Model file for the job. Use its own axes, mm. Face numbers are marked on the shaded views. A direction names the side the tool comes from. Round coordinates to 2 decimals unless told otherwise and drop trailing zeros. Loops run counter-clockwise (first coordinate to the right, second up) from the corner with the lowest first, then second, coordinate; pieces in that order, holes last. Notation, with made-up numbers: (44.25, -33) -> (48.25, -33) arc R5 ccw to (48.25, -26) -> close; hole circle Ø7 at (36.5, -7.5). An arc over 180 degrees is marked (long way). Use a Markdown table: item, result. Add a question column.
```python
from build123d import *

# Parameters (mm, degrees)
F0_W     = 76.2
F0_H     = 38.1
F0_R     = 3.9040723684
F0_W_2   = 0.6455261652
F0_H_2   = 4.2599751749
F0_H_3   = 6.0485428542
F0_R_2   = 3.8989
F1_DEPTH = 12.7


with BuildPart() as f1:
    # F0 (on Top) → F1 (new body)
    with BuildSketch(Plane.XY):
        Rectangle(F0_W, F0_H)
        Polygon((5.4683112539, -8.3463666961), (4.0425748882, -11.8080461533), (0.725272804, -13.5434007948), (-2.9313924856, -12.7404388974), (-5.2164266525, -9.774875257), (-5.0606368145, -6.0343300593), (-2.5369187683, -3.269045974), (1.1738517643, -2.7729301572), (4.3353640105, -4.7781207134), align=None, mode=Mode.SUBTRACT)
        with Locations((-14.1024813056, 6.9073382765)):
            Circle(F0_R, mode=Mode.SUBTRACT)
        Polygon((-31.2197456793, 14.5646184978), (-32.5964540855, 12.8382807598), (-34.8045229299, 12.8382807598), (-36.1812313362, 14.5646184978), (-35.6898897947, 16.7173264462), (-33.7004885077, 17.6753716126), (-31.7110872208, 16.7173264462), align=None, mode=Mode.SUBTRACT)
        with Locations((-1.035253305, 14.0512490247)):
            Rectangle(F0_W_2, F0_H_2, mode=Mode.SUBTRACT)
        Polygon((-4.533408102, 12.5120609141), (-4.533408102, 11.9212614372), (-7.7013370861, 11.9212614372), (-7.7013370861, 17.60413051), (-4.533408102, 17.60413051), (-4.533408102, 17.0170623983), (-7.0408854604, 17.0170623983), (-7.0408854604, 15.1862059144), (-4.6851502834, 15.1862059144), (-4.6851502834, 14.6028691678), (-7.0408854604, 14.6028691678), (-7.0408854604, 12.5120609141), align=None, mode=Mode.SUBTRACT)
        with Locations((-3.0489466797, 14.9455328644)):
            Rectangle(F0_W_2, F0_H_3, mode=Mode.SUBTRACT)
        with BuildLine():
            add(Edge.make_bspline(
                [(-1.3039115934, 17.0108434565), (-1.412743076, 17.1178092565), (-1.412743076, 17.3354722216)],
                knots=[0, 0, 0, 1, 1, 1], degree=2))
            add(Edge.make_bspline(
                [(-1.412743076, 17.3354722216), (-1.412743076, 17.5568665519), (-1.3039115934, 17.6601009868)],
                knots=[0, 0, 0, 1, 1, 1], degree=2))
            add(Edge.make_bspline(
                [(-1.3039115934, 17.6601009868), (-1.1950801108, 17.7633354217), (-1.0309000457, 17.7633354217)],
                knots=[0, 0, 0, 1, 1, 1], degree=2))
            add(Edge.make_bspline(
                [(-1.0309000457, 17.7633354217), (-0.8754264992, 17.7633354217), (-0.7628636515, 17.6582353042)],
                knots=[0, 0, 0, 1, 1, 1], degree=2))
            add(Edge.make_bspline(
                [(-0.7628636515, 17.6582353042), (-0.6503008038, 17.5531351868), (-0.6503008038, 17.3354722216)],
                knots=[0, 0, 0, 1, 1, 1], degree=2))
            add(Edge.make_bspline(
                [(-0.6503008038, 17.3354722216), (-0.6503008038, 17.1178092565), (-0.7628636515, 17.0108434565)],
                knots=[0, 0, 0, 1, 1, 1], degree=2))
            add(Edge.make_bspline(
                [(-0.7628636515, 17.0108434565), (-0.8754264992, 16.9038776565), (-1.0309000457, 16.9038776565)],
                knots=[0, 0, 0, 1, 1, 1], degree=2))
            add(Edge.make_bspline(
                [(-1.0309000457, 16.9038776565), (-1.1950801108, 16.9038776565), (-1.3039115934, 17.0108434565)],
                knots=[0, 0, 0, 1, 1, 1], degree=2))
        make_face(mode=Mode.SUBTRACT)
        with Locations((13.814676553, 7.1951444261)):
            Circle(F0_R_2, mode=Mode.SUBTRACT)
        with BuildLine():
            Line((3.7539538223, 11.9212614372), (3.275095299, 11.9212614372))
            Line((3.275095299, 11.9212614372), (3.1469850967, 12.5282301629))
            Line((3.1469850967, 12.5282301629), (3.1158903874, 12.5282301629))
            add(Edge.make_bspline(
                [(3.1158903874, 12.5282301629), (2.7974805641, 12.127730307), (2.4809364233, 11.9853165384)],
                knots=[0, 0, 0, 1, 1, 1], degree=2))
            add(Edge.make_bspline(
                [(2.4809364233, 11.9853165384), (2.1643922826, 11.8429027698), (1.6892651244, 11.8429027698)],
                knots=[0, 0, 0, 1, 1, 1], degree=2))
            add(Edge.make_bspline(
                [(1.6892651244, 11.8429027698), (1.0561768429, 11.8429027698), (0.6967220033, 12.1700191117)],
                knots=[0, 0, 0, 1, 1, 1], degree=2))
            add(Edge.make_bspline(
                [(0.6967220033, 12.1700191117), (0.3372671638, 12.4971354536), (0.3372671638, 13.0991290258)],
                knots=[0, 0, 0, 1, 1, 1], degree=2))
            add(Edge.make_bspline(
                [(0.3372671638, 13.0991290258), (0.3372671638, 14.3889375678), (2.4007120733, 14.4511269864)],
                knots=[0, 0, 0, 1, 1, 1], degree=2))
            Line((2.4007120733, 14.4511269864), (3.1233531176, 14.4747589655))
            Line((3.1233531176, 14.4747589655), (3.1233531176, 14.7396858887))
            add(Edge.make_bspline(
                [(3.1233531176, 14.7396858887), (3.1233531176, 15.2409326028), (2.9081777292, 15.4797399702)],
                knots=[0, 0, 0, 1, 1, 1], degree=2))
            add(Edge.make_bspline(
                [(2.9081777292, 15.4797399702), (2.6930023408, 15.7185473377), (2.2178751826, 15.7185473377)],
                knots=[0, 0, 0, 1, 1, 1], degree=2))
            add(Edge.make_bspline(
                [(2.2178751826, 15.7185473377), (1.6855337593, 15.7185473377), (1.0138880383, 15.3926747842)],
                knots=[0, 0, 0, 1, 1, 1], degree=2))
            Line((1.0138880383, 15.3926747842), (0.8148818987, 15.886458768))
            add(Edge.make_bspline(
                [(0.8148818987, 15.886458768), (1.1295603569, 16.056857775), (1.5045625511, 16.153873268)],
                knots=[0, 0, 0, 1, 1, 1], degree=2))
            add(Edge.make_bspline(
                [(1.5045625511, 16.153873268), (1.8795647453, 16.250888761), (2.2576764105, 16.250888761)],
                knots=[0, 0, 0, 1, 1, 1], degree=2))
            add(Edge.make_bspline(
                [(2.2576764105, 16.250888761), (3.0188748943, 16.250888761), (3.3864143583, 15.913200218)],
                knots=[0, 0, 0, 1, 1, 1], degree=2))
            add(Edge.make_bspline(
                [(3.3864143583, 15.913200218), (3.7539538223, 15.5755116749), (3.7539538223, 14.8292386515)],
                knots=[0, 0, 0, 1, 1, 1], degree=2))
            Line((3.7539538223, 14.8292386515), (3.7539538223, 11.9212614372))
        make_face(mode=Mode.SUBTRACT)
        with BuildLine():
            add(Edge.make_bspline(
                [(7.5636776065, 13.7869439956), (7.8298483182, 13.5070916119), (7.8298483182, 13.0829597769)],
                knots=[0, 0, 0, 1, 1, 1], degree=2))
            add(Edge.make_bspline(
                [(7.8298483182, 13.0829597769), (7.8298483182, 12.488428935), (7.3870596577, 12.1656658524)],
                knots=[0, 0, 0, 1, 1, 1], degree=2))
            add(Edge.make_bspline(
                [(7.3870596577, 12.1656658524), (6.9442709971, 11.8429027698), (6.1432712854, 11.8429027698)],
                knots=[0, 0, 0, 1, 1, 1], degree=2))
            add(Edge.make_bspline(
                [(6.1432712854, 11.8429027698), (5.2962514039, 11.8429027698), (4.8223680341, 12.1115610582)],
                knots=[0, 0, 0, 1, 1, 1], degree=2))
            Line((4.8223680341, 12.1115610582), (4.8223680341, 12.7098232652))
            add(Edge.make_bspline(
                [(4.8223680341, 12.7098232652), (5.129583762, 12.5543497187), (5.4809539772, 12.4654188501)],
                knots=[0, 0, 0, 1, 1, 1], degree=2))
            add(Edge.make_bspline(
                [(5.4809539772, 12.4654188501), (5.8323241923, 12.3764879815), (6.1594405342, 12.3764879815)],
                knots=[0, 0, 0, 1, 1, 1], degree=2))
            add(Edge.make_bspline(
                [(6.1594405342, 12.3764879815), (6.6644186134, 12.3764879815), (6.9361863727, 12.5375585757)],
                knots=[0, 0, 0, 1, 1, 1], degree=2))
            add(Edge.make_bspline(
                [(6.9361863727, 12.5375585757), (7.2079541321, 12.6986291699), (7.2079541321, 13.0294768769)],
                knots=[0, 0, 0, 1, 1, 1], degree=2))
            add(Edge.make_bspline(
                [(7.2079541321, 13.0294768769), (7.2079541321, 13.2782345514), (6.9927787437, 13.4548525002)],
                knots=[0, 0, 0, 1, 1, 1], degree=2))
            add(Edge.make_bspline(
                [(6.9927787437, 13.4548525002), (6.7776033553, 13.6314704491), (6.1507340156, 13.8727653933)],
                knots=[0, 0, 0, 1, 1, 1], degree=2))
            add(Edge.make_bspline(
                [(6.1507340156, 13.8727653933), (5.5562031737, 14.0941597236), (5.3055798167, 14.2595835771)],
                knots=[0, 0, 0, 1, 1, 1], degree=2))
            add(Edge.make_bspline(
                [(5.3055798167, 14.2595835771), (5.0549564597, 14.4250074306), (4.932443305, 14.6345857713)],
                knots=[0, 0, 0, 1, 1, 1], degree=2))
            add(Edge.make_bspline(
                [(4.932443305, 14.6345857713), (4.8099301504, 14.844164112), (4.8099301504, 15.1352105911)],
                knots=[0, 0, 0, 1, 1, 1], degree=2))
            add(Edge.make_bspline(
                [(4.8099301504, 15.1352105911), (4.8099301504, 15.6563579191), (5.2340619853, 15.9579765994)],
                knots=[0, 0, 0, 1, 1, 1], degree=2))
            add(Edge.make_bspline(
                [(5.2340619853, 15.9579765994), (5.6581938202, 16.2595952796), (6.395760325, 16.2595952796)],
                knots=[0, 0, 0, 1, 1, 1], degree=2))
            add(Edge.make_bspline(
                [(6.395760325, 16.2595952796), (7.0835752948, 16.2595952796), (7.7415393437, 15.9797428959)],
                knots=[0, 0, 0, 1, 1, 1], degree=2))
            Line((7.7415393437, 15.9797428959), (7.5114384949, 15.4548642028))
            add(Edge.make_bspline(
                [(7.5114384949, 15.4548642028), (6.8708874832, 15.7185473377), (6.3497401552, 15.7185473377)],
                knots=[0, 0, 0, 1, 1, 1], degree=2))
            add(Edge.make_bspline(
                [(6.3497401552, 15.7185473377), (5.8907822458, 15.7185473377), (5.657571926, 15.5748897807)],
                knots=[0, 0, 0, 1, 1, 1], degree=2))
            add(Edge.make_bspline(
                [(5.657571926, 15.5748897807), (5.4243616062, 15.4312322237), (5.4243616062, 15.1787431842)],
                knots=[0, 0, 0, 1, 1, 1], degree=2))
            add(Edge.make_bspline(
                [(5.4243616062, 15.1787431842), (5.4243616062, 15.0071003888), (5.5120486865, 14.8870748109)],
                knots=[0, 0, 0, 1, 1, 1], degree=2))
            add(Edge.make_bspline(
                [(5.5120486865, 14.8870748109), (5.5997357667, 14.7670492329), (5.7937667528, 14.6582177504)],
                knots=[0, 0, 0, 1, 1, 1], degree=2))
            add(Edge.make_bspline(
                [(5.7937667528, 14.6582177504), (5.9877977389, 14.5493862678), (6.5400397762, 14.342917398)],
                knots=[0, 0, 0, 1, 1, 1], degree=2))
            add(Edge.make_bspline(
                [(6.5400397762, 14.342917398), (7.2975068949, 14.0667963794), (7.5636776065, 13.7869439956)],
                knots=[0, 0, 0, 1, 1, 1], degree=2))
        make_face(mode=Mode.SUBTRACT)
    extrude(amount=F1_DEPTH)


solid = f1.part
```
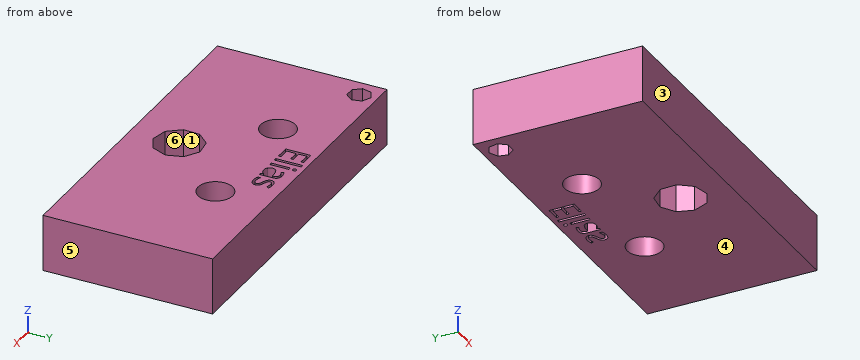
1) Pull direction Y, two halves, no side cores. Call the marked faces 1, 2, 3 and 4: +Y half, -Y half, draft (parallel to the pull), parting line (faces both ways), or undercut.
2) Cut at B-B on y = -11. Write the cut outline in (x, z), and give its area (3 significant figures).
3) Tool access for the marked faces 5 and 6: list every direction of +Z, -Z, +X, -X, +Y, -Y with a clear straight run to the whole face (end or side of a thin tool).
4) Cut at A-A on y = 8.5. Write the cut outline in (x, z), and give its area (3 significant figures).
5) Pin check, flat tips, straight feed: pin 1 Ø4.5 at (x, y) = (-14.1, 6.91) entering from +Z; pin 2 Ø8 at (x, y) = (13, 3.5) entering from -Z. Stop position of each tip, or through.
6) Cut at C-C on z = 8.5. Count the separate pieces of the cut face and the enclosed holes in it, and give its area (3 significant figures).
7) Wall check: probe 1 along X at (y, z) = (7, 5.25); probe 2 along X at (y, z) = (17.5, 2); probe 3 along Y at (x, z) = (-14, 5). Give the ranges that are in metal, low to high. Write a range as from..to.
Established:
| question | item | result |
|---|---|---|
| 1 | face 1 | undercut |
| 1 | face 2 | +Y half |
| 1 | face 3 | -Y half |
| 1 | face 4 | draft |
| 2 | outline | (-38.1, 0) -> (-4.27, 0) -> (-4.27, 12.7) -> (-38.1, 12.7) -> close; (4.38, 0) -> (38.1, 0) -> (38.1, 12.7) -> (4.38, 12.7) -> close |
| 2 | area | 858 mm^2 |
| 3 | face 5 | +Z, -Z, +X, +Y, -Y |
| 3 | face 6 | +Z, -Z |
| 4 | outline | (-38.1, 0) -> (-17.67, 0) -> (-17.67, 12.7) -> (-38.1, 12.7) -> close; (-10.54, 0) -> (10.14, 0) -> (10.14, 12.7) -> (-10.54, 12.7) -> close; (17.49, 0) -> (38.1, 0) -> (38.1, 12.7) -> (17.49, 12.7) -> close |
| 4 | area | 784 mm^2 |
| 5 | pin 1 | passes through |
| 5 | pin 2 | stops at z = 0 |
| 6 | separate pieces | 1 |
| 6 | enclosed holes | 10 |
| 6 | area | 2,670 mm^2 |
| 7 | probe 1 | x = -38.1..-18.01, -10.2..9.92, 17.71..38.1 |
| 7 | probe 2 | x = -38.1..-34.06, -33.34..-7.7, -4.53..-3.37, -2.73..-1.39, -0.67..38.1 |
| 7 | probe 3 | y = -19.05..3, 10.81..19.05 |
